Autodesk Inventor part; units mm, degrees
ref_plane "YZ Plane" through (0, 0, 0) normal (1, 0, 0) x (0, 1, 0)
ref_plane "XZ Plane" through (0, 0, 0) normal (0, 1, 0) x (-1, 0, 0)
ref_plane "XY Plane" through (0, 0, 0) normal (0, 0, 1) x (1, 0, 0)
sketch "Skizze1" plane through (0, 0, 0) normal (0, 0, 1) x (1, 0, 0)
  line L0 (-4.9, 0) -> (4.9, 0)
  line L1 (0, -32.55) -> (0, 32.55)
  line L2 (0, 5) -> (0, -5) construction
  line L3 (0, 19.75) -> (0, -19.75) construction
  line L4 (-3.5, 19.75) -> (-3.5, -19.75)
  line L5 (3.5, -19.75) -> (3.5, 19.75)
  arc A0 (3.5, 19.75) -> (-3.5, 19.75) centre (0, 19.75) ccw
  arc A1 (-3.5, -19.75) -> (3.5, -19.75) centre (0, -19.75) ccw
  line L6 (0, 3.75) -> (0, 13.75) construction
  line L7 (2.5, 3.75) -> (2.5, 13.75)
  line L8 (-2.5, 13.75) -> (-2.5, 3.75)
  arc A2 (-2.5, 3.75) -> (2.5, 3.75) centre (0, 3.75) ccw
  arc A3 (2.5, 13.75) -> (-2.5, 13.75) centre (0, 13.75) ccw
  line L9 (0, -13.75) -> (0, -3.75) construction
  line L10 (2.5, -13.75) -> (2.5, -3.75)
  line L11 (-2.5, -3.75) -> (-2.5, -13.75)
  arc A4 (-2.5, -13.75) -> (2.5, -13.75) centre (0, -13.75) ccw
  arc A5 (2.5, -3.75) -> (-2.5, -3.75) centre (0, -3.75) ccw
  point P0 (0, 0)
  point P1 (0, 0)
  point P2 (0, 0)
  point P3 (0, 8.75)
  point P4 (0, -8.75)
  dimension "d2" = 7
  dimension "d3" = 1.25
  dimension "d4" = 1.25
  dimension "d5" = 23.25
  dimension "d17" = 10
  dimension "d18" = 10
  dimension "d19" = 5
extrude "Extrusion3" add sketch "Skizze1" along normal blind 0.5 contours L4 A0 L1 A3 L8 A2 L0 | L0 L1 A5 L11 A4 A1 L4 | L1 A2 L7 A3 A0 L5 L0 | L0 L5 A1 L1 A4 L10 A5
sketch "Skizze4" plane through (0, 0, 0) normal (0, 0, -1) x (-1, 0, 0)
  line L0 (3.5, 19.75) -> (3.5, -19.75)
  arc A0 (3.5, 19.75) -> (-3.5, 19.75) centre (0, 19.75) ccw
  line L1 (-3.5, -19.75) -> (-3.5, 19.75)
  arc A1 (-3.5, -19.75) -> (3.5, -19.75) centre (0, -19.75) ccw
  point P0 (0, 0)
extrude "Extrusion4" add sketch "Skizze4" along normal blind 1
sketch "Skizze5" plane through (0, 0, 0.5) normal (0, 0, 1) x (1, 0, 0)
  arc A0 (-3.5, -19.75) -> (3.5, -19.75) centre (0, -19.75) ccw
  arc A1 (3.5, 19.75) -> (-3.5, 19.75) centre (0, 19.75) ccw
  point P0 (0, 0)
hole "Bohrung2" at (0, 19.75, 0.5) at (0, -19.75, 0.5) direction (0, 0, -1) diameter 2.4 end through all countersink diameter 4.6 countersink angle 90
sketch "Skizze6" plane through (0, 0, 0) normal (0, 0, 1) x (1, 0, 0)
  arc A0 (-2.5, -13.75) -> (2.5, -13.75) centre (0, -13.75) ccw
  arc A1 (2.5, -3.75) -> (-2.5, -3.75) centre (0, -3.75) ccw
  line L0 (-2.5, -3.75) -> (-2.5, -13.75)
  line L1 (0, -3.75) -> (0, -13.75)
  line L2 (0, -13.75) -> (0, -8.75)
  line L3 (0, -8.75) -> (-1.5, -8.75)
  line L4 (0, -6.75) -> (0, -10.75) construction
  line L5 (2, -6.75) -> (2, -10.75)
  line L6 (-2, -10.75) -> (-2, -6.75)
  arc A2 (2, -6.75) -> (-2, -6.75) centre (0, -6.75) ccw
  arc A3 (-2, -10.75) -> (2, -10.75) centre (0, -10.75) ccw
  point P0 (0, 0)
  dimension "d32" = 8
  dimension "d33" = 4
extrude "Extrusion5" cut sketch "Skizze6" against normal through all
pattern_linear "Rechteckige Anordnung1" count 2 spacing 17.5 along (0, 1, 0) of "Extrusion5"
properties part number "13_1087_019"
Can you work these out from the model? Positions are in its coordinate system, mm. A direction names the side the tool comes from. Coordinates: 2 decimals unless noted, no trailing zeros.
1) For pin 1 (2 mm diameter, centred on x = 0, y = -19.75, fed in from +Z); pin 2 (1.5 mm diameter, centred on x = 0, y = -5, fed in from +Z), each with a flat end and sliding along its axis, tell me the tip position at first contact or that it passes through.
2) Thinking about a two-plate mould opening in X: for faces 4 (the cylindrical face through (-0.05, -18.55, -0.8)), 5 (the flat face through (3.5, 0, 0)), 6 (the flat face through (-3.5, 0, 0)), which applies, pulls with the +X half, pulls with the -X half, needs draft (parallel to the pull), parting line crosses it, or undercut?
3) Which directions (+Z, -Z, +X, -X, +Y, -Y) give clear straight access to the entire face, cutting with the end or side of a thin tool? Please do faces 1 (the flat face through (0, 0, -1)), 2 (the flat face through (-2.2, 8.9, 0)), 3 (the flat face through (-2, 8.7, -0.5)).
4) I need wall thicknesses on probe 1 along Y at (x, z) = (0, -0.75); probe 2 along X at (y, z) = (19.75, -0.85); probe 3 along Z at (x, y) = (-2, 12). Which ranges of each line are inside material? Lowest first, please.
5) Imagine slicing it at A-A on x = 0. State how many separate pieces and enclosed holes the cut face has, plus the area to 3 significant figures.
Completed:
1. pin 1: passes through
1. pin 2: stops at z = 0
2. face 4: undercut
2. face 5: pulls with the +X half
2. face 6: pulls with the -X half
3. face 1: -Z, +X, -X, +Y, -Y
3. face 2: +Z
3. face 3: +Z, -Z
4. probe 1: y = -23.25 to -20.95, -18.55 to -12.75, -4.75 to 4.75, 12.75 to 18.55, 20.95 to 23.25
4. probe 2: x = -3.5 to -1.2, 1.2 to 3.5
4. probe 3: z = -1 to 0
5. separate pieces: 5
5. enclosed holes: 0
5. area: 29.1 mm2
